Autodesk Inventor part; units mm, degrees
ref_plane "Work Plane6" through (-134.9375, 20, -12.7) normal (0.3947, -0.9188, 0) x (0, 0, 1)
ref_plane "Work Plane7" through (-109.8713, -38.3432, -12.7) normal (0.3947, -0.9188, 0) x (0, 0, 1)
ref_plane "YZ Plane" through (0, 0, 0) normal (1, 0, 0) x (0, 1, 0)
sketch "Sketch1" plane through (0, 0, 0) normal (0, 1, 0) x (-1, 0, 0)
  circle A0 centre (0, 0) radius 135
  circle A1 centre (0, 0) radius 110
  dimension "d0" = 270
  dimension "d1" = 220
extrude "Extrusion1" add sketch "Sketch1" along normal mid plane 20
sketch "Sketch3" plane through (0, 10, 0) normal (0, 1, 0) x (1, 0, 0)
  circle A0 centre (0, 0) radius 125
  circle A1 centre (125, 0) radius 2.5
  circle A2 centre (101.1271, 73.4732) radius 2.5
  circle A3 centre (38.6271, 118.8821) radius 2.5
  circle A4 centre (-38.6271, 118.8821) radius 2.5
  circle A5 centre (-101.1271, 73.4732) radius 2.5
  circle A6 centre (-125, 0) radius 2.5
  circle A7 centre (-101.1271, -73.4732) radius 2.5
  circle A8 centre (-38.6271, -118.8821) radius 2.5
  circle A9 centre (38.6271, -118.8821) radius 2.5
  circle A10 centre (101.1271, -73.4732) radius 2.5
  dimension "d7" = 250
  dimension "d8" = 5
  dimension "d11" = 360
hole "Hole1" at (125, 10, 0) at (101.1271, 10, 73.4732) at (38.6271, 10, 118.8821) at (-38.6271, 10, 118.8821) at (-101.1271, 10, 73.4732) at (-125, 10, 0) at (-101.1271, 10, -73.4732) at (-38.6271, 10, -118.8821) at (38.6271, 10, -118.8821) at (101.1271, 10, -73.4732) direction (0, -1, 0) diameter 5 end through all
ref_plane "Work Plane6" through (-134.9375, 20, -12.7) normal (0.3947, -0.9188, 0) x (0, 0, 1)
ref_plane "Work Plane7" through (-109.8713, -38.3432, -12.7) normal (0.3947, -0.9188, 0) x (0, 0, 1)
sketch "Sketch5" plane through (-109.8713, -38.3432, -12.7) normal (0.3947, -0.9188, 0) x (0, 0, 1)
  circle A0 centre (12.7, -30.2265) radius 20
  point P0 (12.7, -116.0845)
  dimension "d26" = 40
  dimension "d27" = 85.858
extrude "Extrusion4" cut sketch "Sketch5" against normal blind 251.3
properties part number "Cylinder Spacer (x3)"
Build history of the part. All positions in model axes, mm. A direction names the side the tool comes from. Round coordinates to 2 decimals unless told otherwise and drop trailing zeros. Write each loop counter-clockwise with the first axis right and the second up, starting at its lowest first coordinate (ties: lowest second). Pieces come first, ordered by that corner, then holes. Notation, with made-up numbers: (-9.75, 73.5) -> (9.25, 73.5) arc R9 cw to (9.25, 83.5) -> close; hole circle Ø9 at (46, -9.75). An arc over 180 degrees is marked (long way). Use one line per item in the form item = value.
Q1. Band-saw the part on A-A, the plane x = 0. Write the cut outline in (y, z), then the cut area to 3 significant figures.
Conclusion:
outline = (-10, -135) -> (10, -135) -> (10, -110) -> (-10, -110) -> close; (-10, 110) -> (10, 110) -> (10, 135) -> (-10, 135) -> close
area = 1,000 mm²
Q2. Tool access for faces 1 (the cylindrical face through (-116.04, 1.93, 0.29)), 2 (the flat face through (1, 10, 111)): list every direction of +Z, -Z, +X, -X, +Y, -Y with a clear straight run to the whole face (end or side of a thin tool).
Conclusion:
face_1 = +Y
face_2 = +Z, -Z, +X, -X, +Y
Q3. Two-plate mould, pull along Z, no slides. Class faces 3 (the flat face through (-9, -10, 111)), 4 (the cylindrical face through (109.9, -0.1, -4.7)), 5 (the cylindrical face through (107.13, -0.14, 82.15)): released by +Z, released by -Z, zero draft, split by the parting line, or undercut.
Conclusion:
face_3 = zero draft
face_4 = undercut
face_5 = split by the parting line
Q4. Drop flat-ended pins along their axis: P1, Ø8, axis at y = 2, z = -82, coming from the +X side; P2, Ø5, axis at y = -3.5, z = 90.5, coming from the +X side; P3, Ø1, axis at y = -1, z = -101, coming from the -X side; P4, Ø8, axis at x = -38.63, z = -118.88, coming from the -Y side. Give the stop position or say it passes through.
Conclusion:
P1 = 110.19
P2 = 102.38
P3 = -90.14
P4 = -10
Q5. Band-saw the part on B-B, the plane z = 49. Write the cut outline in (x, y).
Conclusion:
outline = (-125.79, -10) -> (-98.48, -10) -> (-98.48, 10) -> (-125.79, 10) -> close; (98.48, -10) -> (125.79, -10) -> (125.79, 10) -> (98.48, 10) -> close
Q6. Band-saw the part on C-C, the plane y = 6. State how many separate pieces and enclosed holes the cut face has, then the cut area to 3 significant figures.
Conclusion:
separate_pieces = 1
enclosed_holes = 11
area = 18,900 mm²
Q7. Drill centre lines: L1, parallel to Z at x = 0, y = 4.5; L2, parallel to Z at x = 33, y = 3.5; L3, parallel to X at y = 7.5, z = -51.5. Where is each one in solid material? Low to high.
Conclusion:
L1 = -135 to -110, 110 to 135
L2 = -130.9 to -104.93, 104.93 to 130.9
L3 = -124.79 to -97.2, 97.2 to 124.79
